```python
from build123d import *
from build123d.topology import SkipClean

# Parameters (mm, degrees)
SKETCH_1_R          = 1.5000000000000002
SKETCH_1_R_2        = 1.5000000000000007
SKETCH_1_R_3        = 3.5000000000000036
SKETCH_1_R_4        = 1.5000000000000004
SKETCH_1_R_5        = 1.5000000000000009
EXTRUDE_1_DEPTH     = 3
EXTRUDE_START       = 7
SKETCH_2_R          = 15.00000000000001
SKETCH_2_R_2        = 1.5000000000000002
SKETCH_2_R_3        = 3.5000000000000036
SKETCH_2_R_4        = 1.5000000000000009
SKETCH_2_R_5        = 1.5000000000000007
EXTRUDE_2_DEPTH     = 7
EXTRUDE_START_2     = 9
SKETCH_6_R          = 22
SKETCH_6_R_2        = 15
EXTRUDE_3_DEPTH     = 9
SKETCH_8_R          = 32
SKETCH_8_R_2        = 12.000000000000002
EXTRUDE_5_DEPTH     = 2
FILLET_1_R          = 10
SKETCH_11_R         = 10
CUT_EXTRUDE_1_DEPTH = 2


with BuildPart() as part:
    # 草图1 → 凸台-拉伸1 (new body)
    with BuildSketch(Plane(origin=(0, 0, 0), x_dir=(1, 0, 0), z_dir=(0, 1, 0))):
        Polygon((-35.00000000000001, -35), (34.99999999999999, -35), (34.99999999999999, 34.99999999999999), (-35.00000000000001, 35), align=None)
        with Locations(Location((4.3e-16, 6.999999999999999, 0), (0, 0, 270))):
            Circle(SKETCH_1_R, mode=Mode.SUBTRACT)
        with Locations(Location((6.999999999999999, -4.3e-16, 0), (0, 0, 270))):
            Circle(SKETCH_1_R_2, mode=Mode.SUBTRACT)
        with Locations(Location((-4.21e-15, 2.73e-15, 0), (0, 0, 270))):
            Circle(SKETCH_1_R_3, mode=Mode.SUBTRACT)
        with Locations(Location((-9.8e-16, -6.999999999999999, 0), (0, 0, 90))):
            Circle(SKETCH_1_R_4, mode=Mode.SUBTRACT)
        with Locations(Location((-6.999999999999999, 1.89e-15, 0), (0, 0, 90))):
            Circle(SKETCH_1_R_2, mode=Mode.SUBTRACT)
        with Locations(Location((25, 25, 0), (0, 0, 270))):
            Circle(SKETCH_1_R_5, mode=Mode.SUBTRACT)
        with Locations(Location((-25, 25, 0), (0, 0, 90))):
            Circle(SKETCH_1_R_5, mode=Mode.SUBTRACT)
        with Locations(Location((25, -25, 0), (0, 0, 270))):
            Circle(SKETCH_1_R_5, mode=Mode.SUBTRACT)
        with Locations(Location((-25, -25, 0), (0, 0, 90))):
            Circle(SKETCH_1_R_5, mode=Mode.SUBTRACT)
    extrude(amount=EXTRUDE_1_DEPTH)

    # 草图2 → 凸台-拉伸2 (add)
    with SkipClean():  # the faces are left unmerged after this step: merging them gives an invalid solid
        with BuildSketch(Plane.XZ.offset(EXTRUDE_START)):
            with Locations(Location((-4.21e-15, -2.73e-15, 0), (0, 0, 270))):
                Circle(SKETCH_2_R)
            with Locations(Location((-9.8e-16, 6.999999999999999, 0), (0, 0, 270))):
                Circle(SKETCH_2_R_2, mode=Mode.SUBTRACT)
            with Locations(Location((-4.21e-15, -2.73e-15, 0), (0, 0, 270))):
                Circle(SKETCH_2_R_3, mode=Mode.SUBTRACT)
            with Locations(Location((-6.999999999999999, -1.89e-15, 0), (0, 0, 270))):
                Circle(SKETCH_2_R_4, mode=Mode.SUBTRACT)
            with Locations(Location((4.3e-16, -6.999999999999999, 0), (0, 0, 270))):
                Circle(SKETCH_2_R_2, mode=Mode.SUBTRACT)
            with Locations(Location((6.999999999999999, 4.3e-16, 0), (0, 0, 270))):
                Circle(SKETCH_2_R_5, mode=Mode.SUBTRACT)
        extrude(amount=-EXTRUDE_2_DEPTH)

    # 草图6 → 凸台-拉伸3 (add)
    with SkipClean():  # the faces are left unmerged after this step: merging them gives an invalid solid
        with BuildSketch(Plane.XZ.offset(EXTRUDE_START_2)):
            with Locations(Location((0, 0, 0), (0, 0, 270))):
                Circle(SKETCH_6_R)
            with Locations(Location((0, 0, 0), (0, 0, 270))):
                Circle(SKETCH_6_R_2, mode=Mode.SUBTRACT)
        extrude(amount=-EXTRUDE_3_DEPTH)

    # 草图8 → 凸台-拉伸5 (add)
    with SkipClean():  # the faces are left unmerged after this step: merging them gives an invalid solid
        with BuildSketch(Plane.XZ):
            with Locations(Location((0, 0, 0), (0, 0, 270))):
                Circle(SKETCH_8_R)
            Circle(SKETCH_8_R_2, mode=Mode.SUBTRACT)
        extrude(amount=EXTRUDE_5_DEPTH)

    # 圆角1
    fillet_1_edges = [part.edges().sort_by_distance(p)[0] for p in [
        (34.99999999999999, 1.5, 35),
        (-35.00000000000001, 1.5, 35),
        (-35.00000000000001, 1.5, -35),
        (34.99999999999999, 1.5, -34.99999999999999),
    ]]
    fillet(fillet_1_edges, radius=FILLET_1_R)

    # 草图11 → 切除-拉伸1 (cut)
    with BuildSketch(Plane(origin=(0, 3, 0), x_dir=(1, 0, 0), z_dir=(0, 1, 0))):
        with Locations(Location((0, 0, 0), (0, 0, 270))):
            Circle(SKETCH_11_R)
    extrude(amount=-CUT_EXTRUDE_1_DEPTH, mode=Mode.SUBTRACT)


solid = part.part
```
Could you check a few things on this model? Use its own coordinates, in mm. A direction names the side the tool comes from. Give positions to 0.01 mm unless a question says otherwise; leave off trailing zeros. Loops run counter-clockwise (first coordinate to the right, second up) from the corner with the lowest first, then second, coordinate; pieces in that order, holes last. Notation, with made-up numbers: (-34.75, 60) - (-9.75, 60) arc R27 ccw to (-9.75, 81) - close; hole circle Ø2 at (-20, 61.25). An arc over 180 degrees is marked (long way). Answer in a Markdown table with one row per item. Add a question column.
Q1. Which directions (+Z, -Z, +X, -X, +Y, -Y) give clear straight access to the entire face, cutting with the end or side of a thin tool? Please do faces 5 (the face through (4, -7, 0)), 6 (the face through (31.99, 1.52, 32.15)).
Q2. For pin 1 (6 mm diameter, centred on y = -4, z = 11, fed in from +X); pin 2 (6 mm diameter, centred on x = 7.5, y = -7.5, fed in from +Z); pin 3 (2.5 mm diameter, centred on x = -7, z = 0, fed in from +Y) (3 decimals); pin 4 (1.5 mm diameter, centred on y = -4.5, z = 11.5, fed in from +X), each with a flat end and sliding along its axis, tell me the tip position at first contact or that it passes through.
Q3. Please list where these lines run through material, in increasing order: L1, parallel to Z at x = -25, y = 1.2; L2, parallel to Z at x = 7, y = 0.75. Write a range as from..to.
Q4. We'd pull the mould along X, two halves only. Please class faces 1 (the face through (0, 1, 35)), 2 (the face through (-9.76, 2.01, -2.17)), 3 (the face through (-21.477, -5.549, 4.769)), 4 (the face through (35, 1, 0)): +X half, -X half, draft (parallel to the pull), parting line (faces both ways), or undercut.
Q5. If we section it at D-D (z = 21): List the corners of the cut face in (x, y) for me.
Q6. If we section it at A-A (z = 0): State how many separate pieces and enclosed holes the cut face has, plus the area to 3 significant figures.
Q7. If we section it at B-B (y = -4.75): List the corners of the cut face in (x, z) for me.
Q8. If we section it at C-C (x = -7): List the corners of the cut face in (y, z) for me, plus the area to 3 significant figures.
The answers:
| question | item | result |
|---|---|---|
| 1 | face 5 | -Y |
| 1 | face 6 | +Z, +X, +Y, -Y |
| 2 | pin 1 | stops at x = 30.78 |
| 2 | pin 2 | stops at z = 21.53 |
| 2 | pin 3 | passes through |
| 2 | pin 4 | stops at x = 19.19 |
| 3 | L1 | z = -35..-26.5, -23.5..23.5, 26.5..35 |
| 3 | L2 | z = -35..-1.5, 1.5..35 |
| 4 | face 1 | draft |
| 4 | face 2 | undercut |
| 4 | face 3 | parting line |
| 4 | face 4 | +X half |
| 5 | outline | (-35, 0) - (-24.15, 0) - (-24.15, -2) - (-6.56, -2) - (-6.56, -9) - (6.56, -9) - (6.56, -2) - (24.15, -2) - (24.15, 0) - (35, 0) - (35, 3) - (-35, 3) - close |
| 6 | separate pieces | 4 |
| 6 | enclosed holes | 0 |
| 6 | area | 442 mm^2 |
| 7 | outline | circle Ø44 at (0, 0); hole circle Ø3 at (-7, 0); hole circle Ø7 at (0, 0); hole circle Ø3 at (0, -7); hole circle Ø3 at (0, 7); hole circle Ø3 at (7, 0) |
| 8 | outline | (-9, -20.86) - (-2, -20.86) - (-2, -31.22) - (0, -31.22) - (0, -35) - (3, -35) - (3, -7.14) - (1, -7.14) - (1, -1.5) - (-7, -1.5) - (-7, -13.27) - (-9, -13.27) - close; (-9, 13.27) - (-7, 13.27) - (-7, 1.5) - (1, 1.5) - (1, 7.14) - (3, 7.14) - (3, 35) - (0, 35) - (0, 31.22) - (-2, 31.22) - (-2, 20.86) - (-9, 20.86) - close |
| 8 | area | 521 mm^2 |
